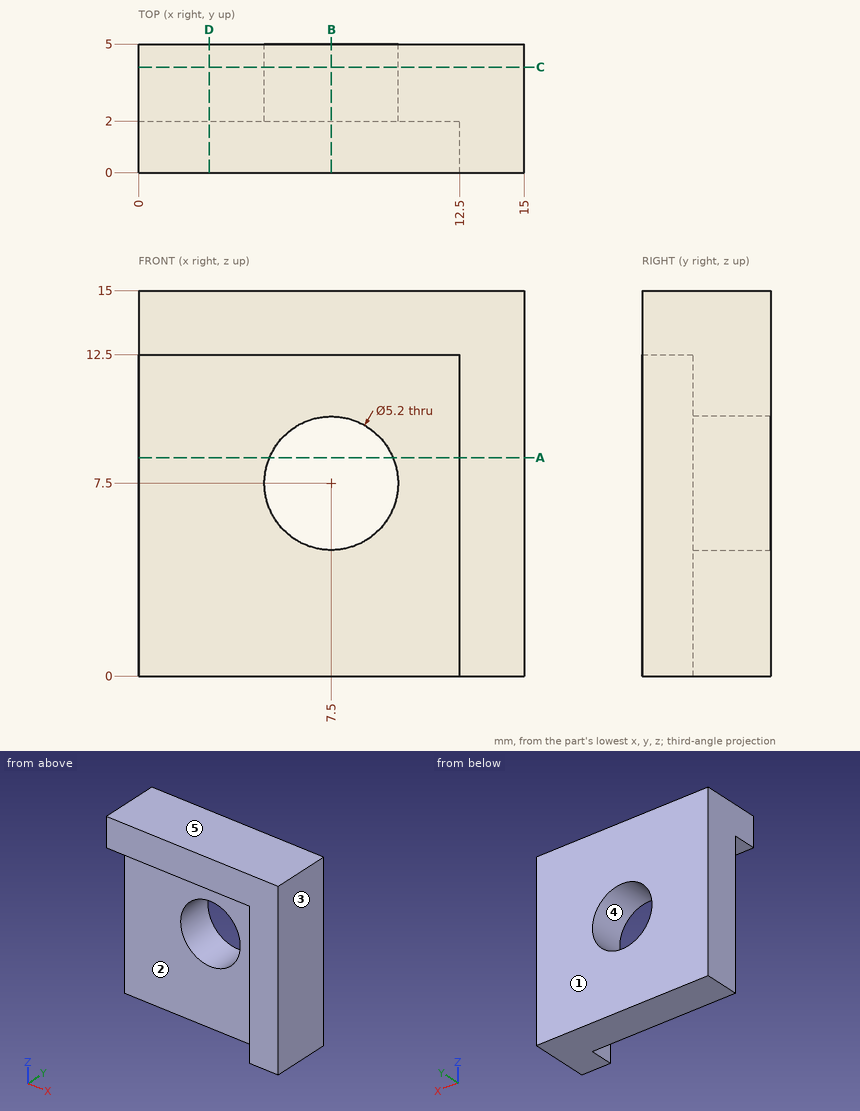
The drawing under review shows one solid part. Ordinate dimensions are in mm from its lowest x, y, z. A direction names the side the tool comes from. Coordinates: 2 decimals unless noted, no trailing zeros. Order: outer loops, then holes, each group sorted by start corner. A loop starts at its lowest first (then second) coordinate and runs counter-clockwise, first axis right, second up. Notation, with made-up numbers: (15, 35.5) -> (60, 35.5) arc R19 ccw to (60, 47.5) -> close; hole circle Ø8 at (38, 55). An arc over 180 degrees is marked (long way). Return JSON: item names as keys, results as strings.
1. We need section D-D on x = 2.75. Write out the cut boundary in (y, z).
Answer block:
{"outline": "(0, 12.5) -> (2, 12.5) -> (2, 0) -> (5, 0) -> (5, 15) -> (0, 15) -> close"}
2. For pin 1 Ø0.6 at (y, z) = (1.5, 5.5) entering from -X; pin 2 Ø6 at (x, z) = (7.5, 7.5) entering from -Y; pin 3 Ø1.6 at (x, y) = (6, 1) entering from -Z, all flat-tipped, find the tip position at first contact; note any pin that passes through.
Answer block:
{"pin 1": "x = 12.5", "pin 2": "y = 2", "pin 3": "z = 12.5"}
3. We need section C-C on y = 4.1. Write out the cut boundary in (x, z).
Answer block:
{"outline": "(0, 0) -> (15, 0) -> (15, 15) -> (0, 15) -> close; hole circle Ø5.2 at (7.5, 7.5)"}
4. For line 1 (X direction, y = 3.9, z = 7.5); line 2 (X direction, y = 0.6, z = 3.5); line 3 (Y direction, x = 0.75, z = 10.5), list the stretches that pass through material, from the lowest coordinate up. Write a range as from..to.
Answer block:
{"line 1": "0..4.9, 10.1..15", "line 2": "12.5..15", "line 3": "2..5"}
5. We need section B-B on x = 7.5. Write out the cut boundary in (y, z).
Answer block:
{"outline": "(0, 12.5) -> (2, 12.5) -> (2, 10.1) -> (5, 10.1) -> (5, 15) -> (0, 15) -> close; (2, 0) -> (5, 0) -> (5, 4.9) -> (2, 4.9) -> close"}
6. The part is to be moulded in two halves that separate along X. For the marked faces 3, 4 and 5, say which applies: +X half, -X half, draft (parallel to the pull), parting line (faces both ways), or undercut.
Answer block:
{"face 3": "+X half", "face 4": "undercut", "face 5": "draft"}
7. We need section A-A on z = 8.5. Write out the cut boundary in (x, y), and give its area (3 significant figures).
Answer block:
{"outline": "(0, 2) -> (5.1, 2) -> (5.1, 5) -> (0, 5) -> close; (9.9, 2) -> (12.5, 2) -> (12.5, 0) -> (15, 0) -> (15, 5) -> (9.9, 5) -> close", "area": "35.6 mm²"}
8. Machinability: for the marked faces 1 and 2, which of the approach directions +Z, -Z, +X, -X, +Y, -Y give a long, thin tool a straight path to every point of the face, cutting with its end or side? Answer none if there is none.
Answer block:
{"face 1": "+Z, -Z, +X, -X, +Y", "face 2": "-Z, -X, -Y"}
